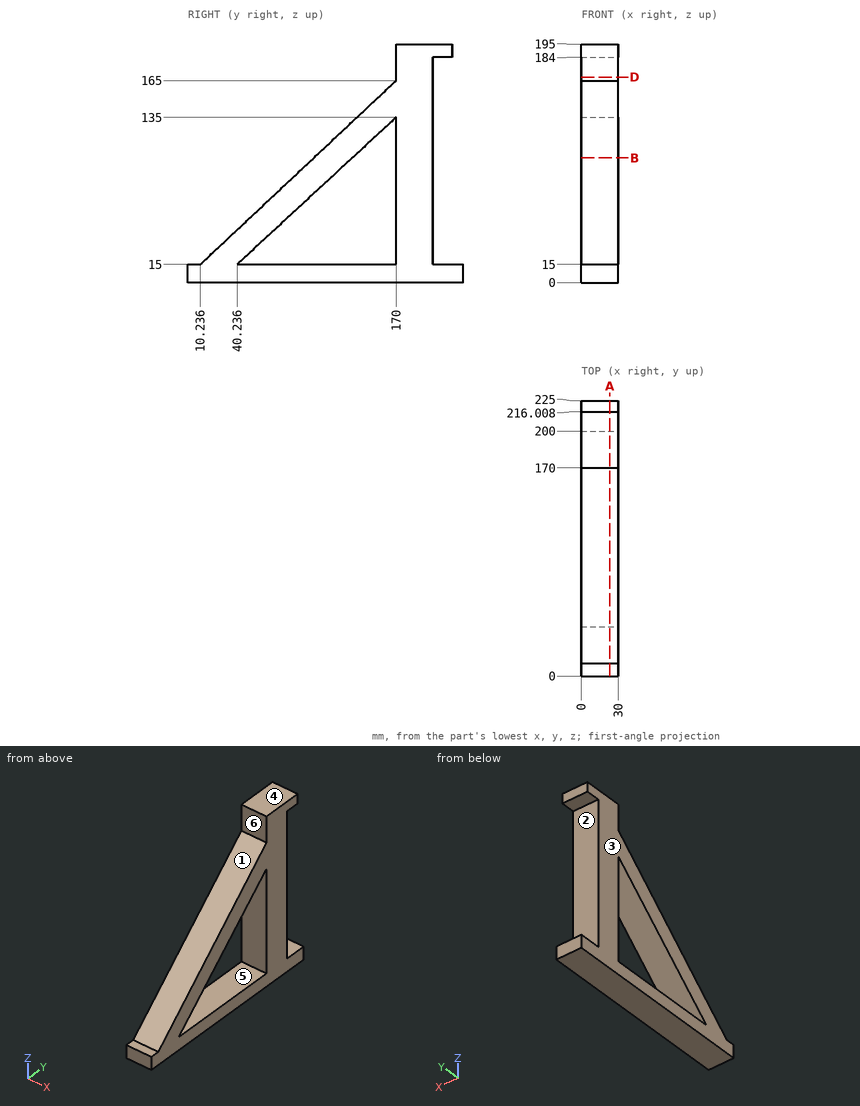
Geometry: see drawing. Coordinates: mm, zero at the bounding-box minimum. A direction names the side the tool comes from. Round coordinates to 2 decimals unless told otherwise and drop trailing zeros. Write each loop counter-clockwise with the first axis right and the second up, starting at its lowest first coordinate (ties: lowest second). Pieces come first, ordered by that corner, then holes. Notation, with made-up numbers: M -16,79 L 30,79 A20 ccw 30,85 Z; hole C 37,16.5 d3. An arc over 180 degrees is marked long. Answer in a Markdown table with one row per item. Add a question column.
(1) Cut plane D-D, the plane z = 168. Return the cut outline in (x, y), then the cut area to 3 significant figures.
(2) Reachability of the marked faces 4, 5 and 6 from +Z, -Z, +X, -X, +Y, -Y: full face, straight path, thin tool, end or side. Return the list, or none.
(3) Cut plane B-B, the plane z = 102. Return the cut outline in (x, y) (1 decimal), then the cut area to 3 significant figures.
(4) Ray query, L1, parallel to Y at x = 6, z = 83; L2, parallel to Y at x = 20.25, z = 177; L3, parallel to Y at x = 5.5, z = 41.5. Return the intervals inside material, ascending.
(5) Draft query along Z for the marked faces 1, 2 and 3. Return one class per face: pulls with the +Z half, pulls with the -Z half, needs draft (parallel to the pull), parting line crosses it, or undercut.
(6) Contact query for flat-ended pins moving along their axis: pin 1 (15 mm diameter, centred on x = 9.5, z = 176.5, fed in from -Y); pin 2 (12 mm diameter, centred on x = 11, z = 191.5, fed in from +Y); pin 3 (2 mm diameter, centred on x = 25, y = 88, fed in from +Z). Output: stop coordinate, or through.
(7) Cut plane A-A, the plane x = 23.25. Return the cut outline in (y, z) (1 decimal).
Established:
| question | item | result |
|---|---|---|
| 1 | outline | M 0,170 L 30,170 L 30,200 L 0,200 Z |
| 1 | area | 900 mm² |
| 2 | face 4 | +Z, +X, -X, +Y, -Y |
| 2 | face 5 | +X, -X |
| 2 | face 6 | +Z, +X, -X, -Y |
| 3 | outline | M 0,102.9 L 30,102.9 L 30,134.3 L 0,134.3 Z; M 0,170 L 30,170 L 30,200 L 0,200 Z |
| 3 | area | 1,840 mm² |
| 4 | L1 | 82.66 to 113.77, 170 to 200 |
| 4 | L2 | 170 to 200 |
| 4 | L3 | 38.46 to 68.89, 170 to 200 |
| 5 | face 1 | pulls with the +Z half |
| 5 | face 2 | undercut |
| 5 | face 3 | needs draft |
| 6 | pin 1 | y = 170 |
| 6 | pin 2 | y = 216.01 |
| 6 | pin 3 | z = 88.95 |
| 7 | outline | M 0,0 L 225,0 L 225,15 L 200,15 L 200,184 L 216,184 L 216,195 L 170,195 L 170,165 L 10.2,15 L 0,15 Z; hole M 40.2,15 L 170,15 L 170,135 Z |
